```python
from build123d import *

# Parameters (mm, degrees)
CROQUIS1_W                      = 200
CROQUIS1_H                      = 150
SALIENTE_EXTRUIR1_DEPTH         = 60
VACIADO1_T                      = 1
CROQUIS3_R                      = 1.7
CORTAR_EXTRUIR2_DEPTH           = 60
CORTAR_EXTRUIR3_DEPTH           = 190
CORTAR_EXTRUIR3_DEPTH_BACK      = 104
CROQUIS4_R                      = 1.7
CORTAR_EXTRUIR4_DEPTH           = 1
TALADRO_DE_MARGEN_PARA_M31_D    = 3.4
CROQUIS14_W                     = 150
CROQUIS14_H                     = 60
CORTAR_EXTRUIR5_DEPTH           = 210
DESPLEGAR_PLIEGUES2_OUTLINE_W   = 202
DESPLEGAR_PLIEGUES2_OUTLINE_H   = 1
DESPLEGAR_PLIEGUES2_DEPTH       = 60
DESPLEGAR_START                 = -1
DESPLEGAR_PLIEGUES2_2_OUTLINE_W = 202
DESPLEGAR_PLIEGUES2_2_OUTLINE_H = 59.141592654
DESPLEGAR_PLIEGUES2_2_OUTLINE_R = 1.7
DESPLEGAR_PLIEGUES2_2_DEPTH     = 1
PROCESAR_START                  = -210.141592654
PROCESAR_PLIEGUES2_OUTLINE_W    = 202
PROCESAR_PLIEGUES2_OUTLINE_H    = 1
PROCESAR_PLIEGUES2_DEPTH        = 59.398442654
PROCESAR_START_2                = 0.74315
PROCESAR_PLIEGUES2_2_OUTLINE_W  = 202
PROCESAR_PLIEGUES2_2_OUTLINE_H  = 1
PROCESAR_PLIEGUES2_2_DEPTH      = 59.398442654
PROCESAR_START_3                = -151
PROCESAR_PLIEGUES2_3_OUTLINE_W  = 202
PROCESAR_PLIEGUES2_3_OUTLINE_H  = 60
PROCESAR_PLIEGUES2_3_OUTLINE_R  = 1.7
PROCESAR_PLIEGUES2_3_DEPTH      = 2.5
PROCESAR_START_4                = -1.5
PROCESAR_PLIEGUES2_4_OUTLINE_W  = 202
PROCESAR_PLIEGUES2_4_OUTLINE_H  = 60
PROCESAR_PLIEGUES2_4_OUTLINE_R  = 1.7
PROCESAR_PLIEGUES2_4_DEPTH      = 2.5
PROCESAR_START_5                = -1
PROCESAR_PLIEGUES2_5_DEPTH      = 202
REDONDEO1_R                     = 2


with BuildPart() as part:
    # Croquis1 → Saliente-Extruir1 (new body)
    with BuildSketch(Plane(origin=(0, 0, 0), x_dir=(1, 0, 0), z_dir=(0, 1, 0))):
        with Locations((100, 75)):
            Rectangle(CROQUIS1_W, CROQUIS1_H)
    extrude(amount=SALIENTE_EXTRUIR1_DEPTH)

    # Vaciado1
    vaciado1_openings = [part.faces().sort_by_distance(p)[0] for p in [
        (100, 60, -75),
    ]]
    offset(amount=VACIADO1_T, openings=vaciado1_openings, kind=Kind.INTERSECTION)

    # Croquis3 → Cortar-Extruir2 (cut)
    with BuildSketch(Plane(origin=(0, 0, 0), x_dir=(-1, 0, 0), z_dir=(0, 1, 0))):
        with Locations(Location((-192.5, -35, 0), (0, 0, 90))):
            Circle(CROQUIS3_R)
        with Locations(Location((-192.5, -115, 0), (0, 0, 90))):
            Circle(CROQUIS3_R)
        with Locations(Location((-7.5, -35, 0), (0, 0, 90))):
            Circle(CROQUIS3_R)
        with Locations(Location((-7.5, -115, 0), (0, 0, 90))):
            Circle(CROQUIS3_R)
    extrude(amount=-CORTAR_EXTRUIR2_DEPTH, mode=Mode.SUBTRACT)

    # Croquis4 → Cortar-Extruir3 (cut, two sides: drawn at the far end of the back side and taken through both)
    with BuildSketch(Plane.XY.offset(-150).offset(-CORTAR_EXTRUIR3_DEPTH_BACK)):
        with Locations((192.5, 25)):
            Circle(CROQUIS4_R)
        with Locations((160, 52.5)):
            Circle(CROQUIS4_R)
        with Locations((120, 52.5)):
            Circle(CROQUIS4_R)
        with Locations((80, 52.5)):
            Circle(CROQUIS4_R)
        with Locations((40, 52.5)):
            Circle(CROQUIS4_R)
        with Locations((7.5, 25)):
            Circle(CROQUIS4_R)
    extrude(amount=CORTAR_EXTRUIR3_DEPTH + CORTAR_EXTRUIR3_DEPTH_BACK, mode=Mode.SUBTRACT)

    # Croquis5 → Cortar-Extruir4 (cut)
    with BuildSketch(Plane(origin=(0, 0, 0), x_dir=(1, 0, 0), z_dir=(0, 1, 0))):
        with BuildLine():
            ThreePointArc((117.1, 76.283509089), (103.304729394, 109.588238483), (70, 123.383509089))
            Line((70, 123.383509089), (70, 29.183509089))
            ThreePointArc((70, 29.183509089), (103.304729394, 42.978779695), (117.1, 76.283509089))
        make_face()
        with BuildLine():
            Line((70, 29.183509089), (70, 123.383509089))
            ThreePointArc((70, 123.383509089), (22.9, 76.283509089), (70, 29.183509089))
        make_face()
    extrude(amount=-CORTAR_EXTRUIR4_DEPTH, mode=Mode.SUBTRACT)

    # Taladro de margen para M31 (through all)
    with Locations(Plane(origin=(0, 0, 0), x_dir=(1, 0, 0), z_dir=(0, 1, 0))):
        with Locations((70, 20.783509089), (70, 131.783509089)):
            Hole(TALADRO_DE_MARGEN_PARA_M31_D / 2)

    # Croquis14 → Cortar-Extruir5 (cut)
    with BuildSketch(Plane(origin=(201, 0, 0), x_dir=(0, 0, -1), z_dir=(1, 0, 0))):
        with Locations((75, 30)):
            Rectangle(CROQUIS14_W, CROQUIS14_H)
    extrude(amount=-CORTAR_EXTRUIR5_DEPTH, mode=Mode.SUBTRACT)

    # Desplegar pliegues2: read off the stored shape, not the designer's step
    # Desplegar pliegues2 outline → Desplegar pliegues2 (cut)
    with BuildSketch(Plane(origin=(0, 0, 0), x_dir=(1, 0, 0), z_dir=(0, 1, 0))):
        with Locations((100, 150.5)):
            Rectangle(DESPLEGAR_PLIEGUES2_OUTLINE_W, DESPLEGAR_PLIEGUES2_OUTLINE_H)
        with Locations((100, -0.5)):
            Rectangle(DESPLEGAR_PLIEGUES2_OUTLINE_W, DESPLEGAR_PLIEGUES2_OUTLINE_H)
    extrude(amount=DESPLEGAR_PLIEGUES2_DEPTH, mode=Mode.SUBTRACT)

    # Desplegar pliegues2 2 outline → Desplegar pliegues2 2 (add)
    # profile 1 of 2: a face of its own
    with BuildSketch(Plane(origin=(0, 0, 0), x_dir=(1, 0, 0), z_dir=(0, 1, 0)).offset(DESPLEGAR_START)):
        with Locations((100, 180.570796327)):
            Rectangle(DESPLEGAR_PLIEGUES2_2_OUTLINE_W, DESPLEGAR_PLIEGUES2_2_OUTLINE_H)
        with Locations((7.5, 175.141592654)):
            Circle(DESPLEGAR_PLIEGUES2_2_OUTLINE_R, mode=Mode.SUBTRACT)
        with Locations((40, 202.641592654)):
            Circle(DESPLEGAR_PLIEGUES2_2_OUTLINE_R, mode=Mode.SUBTRACT)
        with Locations((80, 202.641592654)):
            Circle(DESPLEGAR_PLIEGUES2_2_OUTLINE_R, mode=Mode.SUBTRACT)
        with Locations((120, 202.641592654)):
            Circle(DESPLEGAR_PLIEGUES2_2_OUTLINE_R, mode=Mode.SUBTRACT)
        with Locations((192.5, 175.141592654)):
            Circle(DESPLEGAR_PLIEGUES2_2_OUTLINE_R, mode=Mode.SUBTRACT)
        with Locations((160, 202.641592654)):
            Circle(DESPLEGAR_PLIEGUES2_2_OUTLINE_R, mode=Mode.SUBTRACT)
    # profile 2 of 2: a face of its own
    with BuildSketch(Plane(origin=(0, 0, 0), x_dir=(1, 0, 0), z_dir=(0, 1, 0)).offset(DESPLEGAR_START)):
        with Locations((100, -30.570796327)):
            Rectangle(DESPLEGAR_PLIEGUES2_2_OUTLINE_W, DESPLEGAR_PLIEGUES2_2_OUTLINE_H)
        with Locations((40, -52.641592654)):
            Circle(DESPLEGAR_PLIEGUES2_2_OUTLINE_R, mode=Mode.SUBTRACT)
        with Locations((7.5, -25.141592654)):
            Circle(DESPLEGAR_PLIEGUES2_2_OUTLINE_R, mode=Mode.SUBTRACT)
        with Locations((80, -52.641592654)):
            Circle(DESPLEGAR_PLIEGUES2_2_OUTLINE_R, mode=Mode.SUBTRACT)
        with Locations((120, -52.641592654)):
            Circle(DESPLEGAR_PLIEGUES2_2_OUTLINE_R, mode=Mode.SUBTRACT)
        with Locations((160, -52.641592654)):
            Circle(DESPLEGAR_PLIEGUES2_2_OUTLINE_R, mode=Mode.SUBTRACT)
        with Locations((192.5, -25.141592654)):
            Circle(DESPLEGAR_PLIEGUES2_2_OUTLINE_R, mode=Mode.SUBTRACT)
    extrude(amount=DESPLEGAR_PLIEGUES2_2_DEPTH)

    # Procesar pliegues2: read off the stored shape, not the designer's step
    # Procesar pliegues2 outline → Procesar pliegues2 (cut)
    with BuildSketch(Plane.XY.offset(PROCESAR_START)):
        with Locations((100, -0.5)):
            Rectangle(PROCESAR_PLIEGUES2_OUTLINE_W, PROCESAR_PLIEGUES2_OUTLINE_H)
    extrude(amount=PROCESAR_PLIEGUES2_DEPTH, mode=Mode.SUBTRACT)

    # Procesar pliegues2 2 outline → Procesar pliegues2 2 (cut)
    with BuildSketch(Plane.XY.offset(PROCESAR_START_2)):
        with Locations((100, -0.5)):
            Rectangle(PROCESAR_PLIEGUES2_2_OUTLINE_W, PROCESAR_PLIEGUES2_2_OUTLINE_H)
    extrude(amount=PROCESAR_PLIEGUES2_2_DEPTH, mode=Mode.SUBTRACT)

    # Procesar pliegues2 3 outline → Procesar pliegues2 3 (add)
    with BuildSketch(Plane.XY.offset(PROCESAR_START_3)):
        with Locations((100, 30)):
            Rectangle(PROCESAR_PLIEGUES2_3_OUTLINE_W, PROCESAR_PLIEGUES2_3_OUTLINE_H)
        with Locations((7.5, 25)):
            Circle(PROCESAR_PLIEGUES2_3_OUTLINE_R, mode=Mode.SUBTRACT)
        with Locations((192.5, 25)):
            Circle(PROCESAR_PLIEGUES2_3_OUTLINE_R, mode=Mode.SUBTRACT)
        with Locations((40, 52.5)):
            Circle(PROCESAR_PLIEGUES2_3_OUTLINE_R, mode=Mode.SUBTRACT)
        with Locations((80, 52.5)):
            Circle(PROCESAR_PLIEGUES2_3_OUTLINE_R, mode=Mode.SUBTRACT)
        with Locations((120, 52.5)):
            Circle(PROCESAR_PLIEGUES2_3_OUTLINE_R, mode=Mode.SUBTRACT)
        with Locations((160, 52.5)):
            Circle(PROCESAR_PLIEGUES2_3_OUTLINE_R, mode=Mode.SUBTRACT)
    extrude(amount=PROCESAR_PLIEGUES2_3_DEPTH)

    # Procesar pliegues2 4 outline → Procesar pliegues2 4 (add)
    with BuildSketch(Plane.XY.offset(PROCESAR_START_4)):
        with Locations((100, 30)):
            Rectangle(PROCESAR_PLIEGUES2_4_OUTLINE_W, PROCESAR_PLIEGUES2_4_OUTLINE_H)
        with Locations((7.5, 25)):
            Circle(PROCESAR_PLIEGUES2_4_OUTLINE_R, mode=Mode.SUBTRACT)
        with Locations((192.5, 25)):
            Circle(PROCESAR_PLIEGUES2_4_OUTLINE_R, mode=Mode.SUBTRACT)
        with Locations((40, 52.5)):
            Circle(PROCESAR_PLIEGUES2_4_OUTLINE_R, mode=Mode.SUBTRACT)
        with Locations((80, 52.5)):
            Circle(PROCESAR_PLIEGUES2_4_OUTLINE_R, mode=Mode.SUBTRACT)
        with Locations((120, 52.5)):
            Circle(PROCESAR_PLIEGUES2_4_OUTLINE_R, mode=Mode.SUBTRACT)
        with Locations((160, 52.5)):
            Circle(PROCESAR_PLIEGUES2_4_OUTLINE_R, mode=Mode.SUBTRACT)
    extrude(amount=PROCESAR_PLIEGUES2_4_DEPTH)

    # Procesar pliegues2 5 outline → Procesar pliegues2 5 (cut)
    with BuildSketch(Plane.YZ.offset(PROCESAR_START_5)):
        with BuildLine():
            Line((1.5, -150), (60, -150))
            Line((60, -150), (60, -148.5))
            Line((60, -148.5), (0, -148.5))
            ThreePointArc((0, -148.5), (0.439339828, -149.560660172), (1.5, -150))
        make_face()
        with BuildLine():
            ThreePointArc((1.5, -151), (-0.267766953, -150.267766953), (-1, -148.5))
            Line((-1, -148.5), (-1, -150.74315))
            Line((-1, -150.74315), (0, -150.74315))
            Line((0, -150.74315), (0, -151))
            Line((0, -151), (1.5, -151))
        make_face()
        with BuildLine():
            ThreePointArc((-1, -1.5), (-0.267766953, 0.267766953), (1.5, 1))
            Line((1.5, 1), (0, 1))
            Line((0, 1), (0, 0.74315))
            Line((0, 0.74315), (-1, 0.74315))
            Line((-1, 0.74315), (-1, -1.5))
        make_face()
        with BuildLine():
            Line((60, 0), (1.5, 0))
            ThreePointArc((1.5, 0), (0.439339828, -0.439339828), (0, -1.5))
            Line((0, -1.5), (60, -1.5))
            Line((60, -1.5), (60, 0))
        make_face()
    extrude(amount=PROCESAR_PLIEGUES2_5_DEPTH, mode=Mode.SUBTRACT)

    # Redondeo1
    redondeo1_edges = [part.edges().sort_by_distance(p)[0] for p in [
        (201, 60, -150.5),
        (-1, 60, -150.5),
        (-1, 60, 0.5),
        (201, 60, 0.5),
    ]]
    fillet(redondeo1_edges, radius=REDONDEO1_R)


solid = part.part
```
Source: CAD feature listing. Evaluate the final solid. Frame: model axes, mm. A direction names the side the tool comes from. Coordinates: 2 decimals unless noted, no trailing zeros. Loops run counter-clockwise (first coordinate to the right, second up) from the corner with the lowest first, then second, coordinate; pieces in that order, holes last. Notation, with made-up numbers: M 47,52 L 51,52 A34 ccw 51,87 Z; hole C 14,61.5 d9. An arc over 180 degrees is marked long. Use a Markdown table: item, result. Add a question column.
Q1. Access query for faces 4 (the flat face through (99, 31, 1)), 5 (the flat face through (99, 30, -150)). Directions: +Z, -Z, +X, -X, +Y, -Y. A direction counts if a zero-diameter tool reaches every point of the face in a straight line with its end or side. Return the directions, or none.
Q2. Section query B-B, the plane x = 96.5. Return loops of the section in (y, z).
Q3. Section query C-C, the plane z = -45. Return loops of the section in (x, y).
Q4. First-contact query: pin 1 (3 mm diameter, centred on x = 104.5, z = -117.5, fed in from +Y); pin 2 (8 mm diameter, centred on y = 7, z = -129.5, fed in from -X). Flat tips, straight axial feed; report the tip coordinate or a pass-through.
Q5. Material intervals for L1, parallel to X at y = 52.5, z = -150.35; L2, parallel to X at y = 25, z = 0.6; L3, parallel to Z at x = 49.5, y = 30.5, sorted ascending.
Q6. Draft query along Z for faces 1 (the flat face through (121, 0, -76)), 2 (the flat face through (99, 31, -151)), 3 (the flat face through (121, -1, -76)). Return one class per face: pulls with the +Z half, pulls with the -Z half, needs draft (parallel to the pull), parting line crosses it, or undercut.
Q7. Section query D-D, the plane x = 129.5. Return loops of the section in (y, z), and give its area (3 significant figures).
Q8. Section query A-A, the plane y = 13. Return loops of the section in (x, z).
Result:
| question | item | result |
|---|---|---|
| 1 | face 4 | +Z, +X, -X, +Y, -Y |
| 1 | face 5 | +X, -X, +Y |
| 2 | outline | M -1,-148.5 A2.5 ccw 1.5,-151 L 60,-151 L 60,-150 L 1.5,-150 A1.5 cw 0,-148.5 L 0,-115.22 L -1,-115.22 Z; M -1,-37.35 L 0,-37.35 L 0,-1.5 A1.5 cw 1.5,0 L 60,0 L 60,1 L 1.5,1 A2.5 ccw -1,-1.5 Z |
| 3 | outline | M -1,-1 L 34.79,-1 L 34.79,0 L -1,0 Z; M 105.21,-1 L 201,-1 L 201,0 L 105.21,0 Z |
| 4 | pin 1 | stops at y = 0 |
| 4 | pin 2 | passes through |
| 5 | L1 | x = -1 to 38.3, 41.7 to 78.3, 81.7 to 118.3, 121.7 to 158.3, 161.7 to 201 |
| 5 | L2 | x = -1 to 5.8, 9.2 to 190.8, 194.2 to 201 |
| 5 | L3 | z = -151 to -150, 0 to 1 |
| 6 | face 1 | undercut |
| 6 | face 2 | pulls with the -Z half |
| 6 | face 3 | needs draft |
| 7 | outline | M -1,-148.5 A2.5 ccw 1.5,-151 L 60,-151 L 60,-150 L 1.5,-150 A1.5 cw 0,-148.5 L 0,-1.5 A1.5 cw 1.5,0 L 60,0 L 60,1 L 1.5,1 A2.5 ccw -1,-1.5 Z |
| 7 | area | 270 mm2 |
| 8 | outline | M -1,-151 L 201,-151 L 201,-150 L -1,-150 Z; M -1,0 L 201,0 L 201,1 L -1,1 Z |
